Model file for the job. Use its own axes, mm. A direction names the side the tool comes from. Give positions to 0.01 mm unless a question says otherwise; leave off trailing zeros. Write each loop counter-clockwise with the first axis right and the second up, starting at its lowest first coordinate (ties: lowest second). Pieces come first, ordered by that corner, then holes. Notation, with made-up numbers: (2.5, -38.5) - (48.5, -38.5) arc R10 ccw to (48.5, -26.5) - close; hole circle Ø1 at (20, 47.25). An arc over 180 degrees is marked (long way). Use a Markdown table: item, result. Add a question column.
```python
from build123d import *

# Parameters (mm, degrees)
SKETCH1_W           = 56
SKETCH1_H           = 32
SKETCH1_W_2         = 50
SKETCH1_H_2         = 26
BOSS_EXTRUDE1_DEPTH = 3
SKETCH2_W           = 3
SKETCH2_H           = 3
BOSS_EXTRUDE2_DEPTH = 28
BOSS_EXTRUDE3_DEPTH = 3
BOSS_EXTRUDE4_DEPTH = 3
SKETCH6_W           = 3
SKETCH6_H           = 3
BOSS_EXTRUDE5_DEPTH = 3
SKETCH10_W          = 3
SKETCH10_H          = 26
BOSS_EXTRUDE7_DEPTH = 3
SKETCH10_4_W        = 3
SKETCH10_4_H        = 26
BOSS_EXTRUDE8_DEPTH = 2
SKETCH11_W          = 2
SKETCH11_H          = 6
BOSS_EXTRUDE9_DEPTH = 2


with BuildPart() as part:
    # Sketch1 → Boss-Extrude1 (new body)
    with BuildSketch(Plane(origin=(0, 0, 0), x_dir=(1, 0, 0), z_dir=(0, 1, 0))):
        Rectangle(SKETCH1_W, SKETCH1_H)
        Rectangle(SKETCH1_W_2, SKETCH1_H_2, mode=Mode.SUBTRACT)
    extrude(amount=BOSS_EXTRUDE1_DEPTH)

    # Sketch2 → Boss-Extrude2 (add)
    with BuildSketch(Plane(origin=(0, 0, 0), x_dir=(1, 0, 0), z_dir=(0, 1, 0))):
        with Locations((26.5, 14.5)):
            Rectangle(SKETCH2_W, SKETCH2_H)
        with Locations((26.5, -14.5)):
            Rectangle(SKETCH2_W, SKETCH2_H)
        with Locations((-26.5, -14.5)):
            Rectangle(SKETCH2_W, SKETCH2_H)
        with Locations((-26.5, 14.5)):
            Rectangle(SKETCH2_W, SKETCH2_H)
    extrude(amount=BOSS_EXTRUDE2_DEPTH)

    # Sketch3 → Boss-Extrude3 (add)
    with BuildSketch(Plane.XY.offset(16)):
        Polygon((28, 10), (28, 5), (29.7, 5), (29.7, 8.2), (32.9, 8.2), (32.9, 6.6), (36.1, 6.6), (36.1, 5), (38, 5), (38, 10), align=None)
        Polygon((28, 5), (28, 0), (38, 0), (38, 5), (36.1, 5), (36.1, 3.4), (32.9, 3.4), (32.9, 1.8), (29.7, 1.8), (29.7, 5), align=None)
    boss_extrude3 = extrude(amount=-BOSS_EXTRUDE3_DEPTH)

    # Mirror1: Boss-Extrude3 across plane
    add(boss_extrude3.mirror(Plane.XY))

    # Sketch4 → Boss-Extrude4 (add)
    with BuildSketch(Plane.XY.offset(16)):
        Polygon((5, 0), (0, 0), (-5, 0), (-5, -10), (0, -10), (5, -10), align=None)
        Polygon((1.6, -8.1), (0, -8.1), (-1.6, -8.1), (-1.6, -4.9), (-3.2, -4.9), (-3.2, -1.7), (3.2, -1.7), (3.2, -4.9), (1.6, -4.9), align=None, mode=Mode.SUBTRACT)
    boss_extrude4 = extrude(amount=-BOSS_EXTRUDE4_DEPTH)

    # Mirror2: Boss-Extrude4 across plane
    add(boss_extrude4.mirror(Plane.XY))

    # Sketch6 → Boss-Extrude5 (add)
    # profile 1 of 2: a face of its own
    with BuildSketch(Plane(origin=(0, 28, 0), x_dir=(1, 0, 0), z_dir=(0, 1, 0))):
        with Locations((26.5, -14.5)):
            Rectangle(SKETCH6_W, SKETCH6_H)
    # profile 2 of 2: a face of its own
    with BuildSketch(Plane(origin=(0, 28, 0), x_dir=(1, 0, 0), z_dir=(0, 1, 0))):
        Polygon((-28, -16), (25, -16), (25, -13), (28, -13), (28, 16), (-28, 16), align=None)
        Polygon((25, 6), (25, -13), (-25, -13), (-25, -9), (-25, 6), (-25, 9), (-25, 13), (25, 13), (25, 9), align=None, mode=Mode.SUBTRACT)
    extrude(amount=BOSS_EXTRUDE5_DEPTH)

    # Sketch10 → Boss-Extrude7 (add)
    with BuildSketch(Plane(origin=(0, 3, 0), x_dir=(1, 0, 0), z_dir=(0, 1, 0))):
        with Locations((8, 0)):
            Rectangle(SKETCH10_W, SKETCH10_H)
        with Locations((-8, 0)):
            Rectangle(SKETCH10_W, SKETCH10_H)
    extrude(amount=-BOSS_EXTRUDE7_DEPTH)

    # Sketch10_4 → Boss-Extrude8 (add)
    with BuildSketch(Plane(origin=(0, 3, 0), x_dir=(1, 0, 0), z_dir=(0, 1, 0))):
        with Locations((17, 0)):
            Rectangle(SKETCH10_4_W, SKETCH10_4_H)
        with Locations((-17, 0)):
            Rectangle(SKETCH10_4_W, SKETCH10_4_H)
    extrude(amount=-BOSS_EXTRUDE8_DEPTH)

    # Sketch11 → Boss-Extrude9 (add)
    with BuildSketch(Plane(origin=(0, 31, 0), x_dir=(1, 0, 0), z_dir=(0, 1, 0))):
        Polygon((15, -3), (15, -13), (25, -13), (25, -3), (17, -3), align=None)
        with Locations((16, 0)):
            Rectangle(SKETCH11_W, SKETCH11_H)
        Polygon((15, 13), (15, 3), (17, 3), (25, 3), (25, 13), align=None)
        Polygon((-17, 3), (-15, 3), (-15, 13), (-25, 13), (-25, 3), align=None)
        Polygon((-25, -3), (-25, -13), (-15, -13), (-15, -3), (-17, -3), align=None)
        with Locations((-16, 0)):
            Rectangle(SKETCH11_W, SKETCH11_H)
    extrude(amount=-BOSS_EXTRUDE9_DEPTH)


solid = part.part
```
(1) Probe probe 1 along X at (y, z) = (2, 10); probe 2 along Z at (x, y) = (-2, -1.5); probe 3 along X at (y, z) = (18.5, 14.5). List the from-to ranges inside material, lowest first. Write a range as [from, to].
(2) Band-saw the part on A-A (y = -7). Write the cut outline in (x, z).
(3) Band-saw the part on B-B (x = 21). Write the cut outline in (y, z), then the cut area to 3 significant figures.
(4) Band-saw the part on C-C (z = 14.5). Give the number of separate pieces and of enclosed holes in the cut face, then the cut area to 3 significant figures.
(5) Which spindle directions (+Z, -Z, +X, -X, +Y, -Y) get a long thin tool onto all of the face, cutting with end or side? Do faces 3 (the flat face through (17, 30, 0)), 4 (the flat face through (-17, 1, 0)), 5 (the flat face through (1.6, -6, -15)), 6 (the flat face through (-16.7, 29, -0.2)), 7 (the flat face through (5, -5, 15)). Say none if no direction does.
(6) Band-saw the part on D-D (y = 4.5). Write the cut outline in (x, z).
(7) Flat gauge pins, fed straight in: pin 1 (2.5 mm diameter, centred on y = -6, z = -14.5, fed in from +X); pin 2 (2.5 mm diameter, centred on x = 17.5, z = 2, fed in from -Y); pin 3 (2.5 mm diameter, centred on y = -4, z = -15, fed in from -X). Where does each tip first touch, or does it go through?
(8) Two-plate mould, pull along Z, no slides. Class faces 1 (the flat face through (-15, 30, 0)), 2 (the flat face through (31, 1.8, 15)): +Z half, -Z half, draft (parallel to the pull), parting line (faces both ways), or undercut.
Model answer:
| question | item | result |
|---|---|---|
| 1 | probe 1 | x = [-28, -25], [-18.5, -15.5], [-9.5, -6.5], [6.5, 9.5], [15.5, 18.5], [25, 28] |
| 1 | probe 2 | z = [-16, -13], [13, 16] |
| 1 | probe 3 | x = [-28, -25], [25, 28] |
| 2 | outline | (-5, -16) - (-1.6, -16) - (-1.6, -13) - (-5, -13) - close; (-5, 13) - (-1.6, 13) - (-1.6, 16) - (-5, 16) - close; (1.6, -16) - (5, -16) - (5, -13) - (1.6, -13) - close; (1.6, 13) - (5, 13) - (5, 16) - (1.6, 16) - close |
| 3 | outline | (0, -16) - (3, -16) - (3, -13) - (0, -13) - close; (0, 13) - (3, 13) - (3, 16) - (0, 16) - close; (28, -16) - (31, -16) - (31, -3) - (29, -3) - (29, -13) - (28, -13) - close; (28, 13) - (29, 13) - (29, 3) - (31, 3) - (31, 16) - (28, 16) - close |
| 3 | area | 76.0 mm^2 |
| 4 | separate pieces | 1 |
| 4 | enclosed holes | 3 |
| 4 | area | 625 mm^2 |
| 5 | face 3 | +Y |
| 5 | face 4 | -Y |
| 5 | face 5 | +Z, -Z |
| 5 | face 6 | none |
| 5 | face 7 | +Z, -Z, +X, -Y |
| 6 | outline | (-28, -16) - (-25, -16) - (-25, -13) - (-28, -13) - close; (-28, 13) - (-25, 13) - (-25, 16) - (-28, 16) - close; (25, -16) - (29.7, -16) - (29.7, -13) - (25, -13) - close; (25, 13) - (29.7, 13) - (29.7, 16) - (25, 16) - close; (36.1, -16) - (38, -16) - (38, -13) - (36.1, -13) - close; (36.1, 13) - (38, 13) - (38, 16) - (36.1, 16) - close |
| 7 | pin 1 | stops at x = 5 |
| 7 | pin 2 | stops at y = 1 |
| 7 | pin 3 | stops at x = -5 |
| 8 | face 1 | undercut |
| 8 | face 2 | draft |
